Geometry: final body of the model. Coordinates: model frame, mm. A direction names the side the tool comes from. Round coordinates to 2 decimals unless told otherwise and drop trailing zeros. Loops run counter-clockwise (first coordinate to the right, second up) from the corner with the lowest first, then second, coordinate; pieces in that order, holes last. Notation, with made-up numbers: (-20.5, 34.5) - (14.5, 34.5) arc R25 cw to (14.5, 56.5) - close; hole circle Ø10 at (84.5, 30.25). An arc over 180 degrees is marked (long way). Return JSON: item names as keys, results as strings. Group by question number.
1. Material intervals for probe 1 along Y at (x, z) = (3.6, 0); probe 2 along Y at (x, z) = (48.5, -22); probe 3 along X at (y, z) = (-7.5, 19), sorted ascending.
2. Draft query along Y for faces 4 (the face through (19.365, 19.961, 10.382)), 5 (the face through (46.93, -19.649, -20.777)), 6 (the face through (47, 31, 0)). Return one class per face: +Y half, -Y half, draft (parallel to the pull), parting line (faces both ways), or undercut.
3. Section C-C on z = -23.5. Count the separate pieces of the cut face and the enclosed holes in it, and give its area (3 significant figures).
4. Section B-B on x = 29. Return loops of the section in (y, z).
5. First-contact query: pin 1 Ø2 at (x, z) = (7, 11) entering from +Y; pin 2 Ø4 at (x, z) = (34, -12) entering from -Y; pin 3 Ø7 at (y, z) = (-22, -22) entering from +X; pin 4 Ø4 at (y, z) = (20, -1) entering from -X. Flat tips, straight axial feed; report the tip coordinate or a pass-through.
6. Section A-A on x = 48. Return loops of the section in (y, z).
7. Set-up query: faces 1 (the face through (47.07, 27.99, -28.15)), 2 (the face through (42, -27, 0)), 3 (the face through (52.641, -12.165, -13.267)). Return all of +Z, -Z, +X, -X, +Y, -Y with unobstructed straight access to the full face (end or side cutting, diameter ignored); none if empty.
from build123d import *

# Parameters (mm, degrees)
BOSS_EXTRU_1_START = -10
ESQUISSE2_W        = 62
ESQUISSE2_H        = 62
ESQUISSE2_R        = 16.5
BOSS_EXTRU_1_DEPTH = 10
CONG_1_R           = 10
D_GAGEMENT_M51_D   = 5.3
SYM_TRIE2_COPY_1_D = 5.3
CONG_2_R           = 4
ESQUISSE5_R        = 18
ESQUISSE5_R_2      = 16.5
BOSS_EXTRU_2_DEPTH = 1.5
CHANFREIN1_SIZE    = 0.2
CHANFREIN2_SIZE    = 0.2
CHANFREIN3_SIZE    = 0.2
CHANFREIN4_SIZE    = 0.2


with BuildPart() as part:
    # Esquisse1 → Révolution1 (revolve)
    with BuildSketch(Plane.XY, mode=Mode.PRIVATE) as r_volution1_sk:
        Polygon((0, 15), (0, 22.5), (52, 22.5), (52, 16.5), (15, 16.5), (15, 16), (5, 16), (5, 15), align=None)
    revolve(r_volution1_sk.sketch.rotate(Axis((-138.831140815, 0, 0), (1, 0, 0)), 90), axis=Axis((-138.831140815, 0, 0), (1, 0, 0)))

    # Esquisse2 → Boss.-Extru.1 (add)
    with BuildSketch(Plane(origin=(52, 0, 0), x_dir=(0, 0, -1), z_dir=(1, 0, 0)).offset(BOSS_EXTRU_1_START)):
        Rectangle(ESQUISSE2_W, ESQUISSE2_H)
        with Locations(Location((0, 0, 0), (0, 0, 180))):
            Circle(ESQUISSE2_R, mode=Mode.SUBTRACT)
    extrude(amount=BOSS_EXTRU_1_DEPTH)

    # Congé1
    cong_1_edges = [part.edges().sort_by_distance(p)[0] for p in [
        (47, 31, -31),
        (47, -31, -31),
        (47, -31, 31),
        (47, 31, 31),
    ]]
    fillet(cong_1_edges, radius=CONG_1_R)

    # Dégagement M51 (through all)
    with Locations(Plane(origin=(52, 0, 0), x_dir=(0, 0, -1), z_dir=(1, 0, 0))):
        with Locations((22, 22)):
            d_gagement_m51 = Hole(D_GAGEMENT_M51_D / 2)

    # Symétrie1: Dégagement M51 across plane
    add(d_gagement_m51.mirror(Plane.XY), mode=Mode.SUBTRACT)

    # Symétrie2: Dégagement M51 across plane
    add(d_gagement_m51.mirror(Plane.ZX), mode=Mode.SUBTRACT)

    # Symétrie2 copy 1 (through all)
    with Locations(Plane(origin=(52, 0, 0), x_dir=(0, 0, 1), z_dir=(1, 0, 0))):
        with Locations((22, 22)):
            Hole(SYM_TRIE2_COPY_1_D / 2)

    # Congé2
    cong_2_edges = [part.edges().sort_by_distance(p)[0] for p in [
        (42, 0, -22.5),
    ]]
    fillet(cong_2_edges, radius=CONG_2_R)

    # Esquisse5 → Boss.-Extru.2 (add)
    with BuildSketch(Plane(origin=(52, 0, 0), x_dir=(0, 0, -1), z_dir=(1, 0, 0))):
        with Locations(Location((0, 0, 0), (0, 0, 180))):
            Circle(ESQUISSE5_R)
        with Locations(Location((0, 0, 0), (0, 0, 180))):
            Circle(ESQUISSE5_R_2, mode=Mode.SUBTRACT)
    extrude(amount=BOSS_EXTRU_2_DEPTH)

    # Chanfrein1
    chanfrein1_edges = [part.edges().sort_by_distance(p)[0] for p in [
        (53.5, 0, -18),
    ]]
    chamfer(chanfrein1_edges, length=CHANFREIN1_SIZE)

    # Chanfrein2
    chanfrein2_edges = [part.edges().sort_by_distance(p)[0] for p in [
        (52, 0, 31),
        (52, 0, -31),
        (52, 31, 0),
        (52, -31, 0),
        (52, 28.071067812, 28.071067812),
        (52, 28.071067812, -28.071067812),
        (52, -28.071067812, -28.071067812),
        (52, -28.071067812, 28.071067812),
    ]]
    chamfer(chanfrein2_edges, length=CHANFREIN2_SIZE)

    # Chanfrein3
    chanfrein3_edges = [part.edges().sort_by_distance(p)[0] for p in [
        (42, 0, 31),
        (42, -31, 0),
        (42, 0, -31),
        (42, 31, 0),
        (42, 28.071067812, 28.071067812),
        (42, 28.071067812, -28.071067812),
        (42, -28.071067812, -28.071067812),
        (42, -28.071067812, 28.071067812),
    ]]
    chamfer(chanfrein3_edges, length=CHANFREIN3_SIZE)

    # Chanfrein4
    chanfrein4_edges = [part.edges().sort_by_distance(p)[0] for p in [
        (0, 0, -15),
        (0, 0, -22.5),
    ]]
    chamfer(chanfrein4_edges, length=CHANFREIN4_SIZE)


solid = part.part
Taken from the geometry:
{
 "1": {"probe 1": "-22.5 to -15, 15 to 22.5", "probe 2": "-30.95 to -24.65, -19.35 to 19.35, 24.65 to 30.95", "probe 3": "0 to 52"},
 "2": {"face 4": "parting line", "face 5": "undercut", "face 6": "+Y half"},
 "3": {"separate pieces": "3", "enclosed holes": "0", "area": "543 mm2"},
 "4": {"outline": "circle Ø45 at (0, 0); hole circle Ø33 at (0, 0)"},
 "5": {"pin 1": "y = 20.16", "pin 2": "y = -20.16", "pin 3": "x = 52", "pin 4": "x = 0"},
 "6": {"outline": "(-31, -21) arc R10 ccw to (-21, -31) - (21, -31) arc R10 ccw to (31, -21) - (31, 21) arc R10 ccw to (21, 31) - (-21, 31) arc R10 ccw to (-31, 21) - close; hole circle Ø5.3 at (-22, -22); hole circle Ø5.3 at (-22, 22); hole circle Ø33 at (0, 0); hole circle Ø5.3 at (22, -22); hole circle Ø5.3 at (22, 22)"},
 "7": {"face 1": "-Z, +X, -X, +Y", "face 2": "-X", "face 3": "+X"}
}
